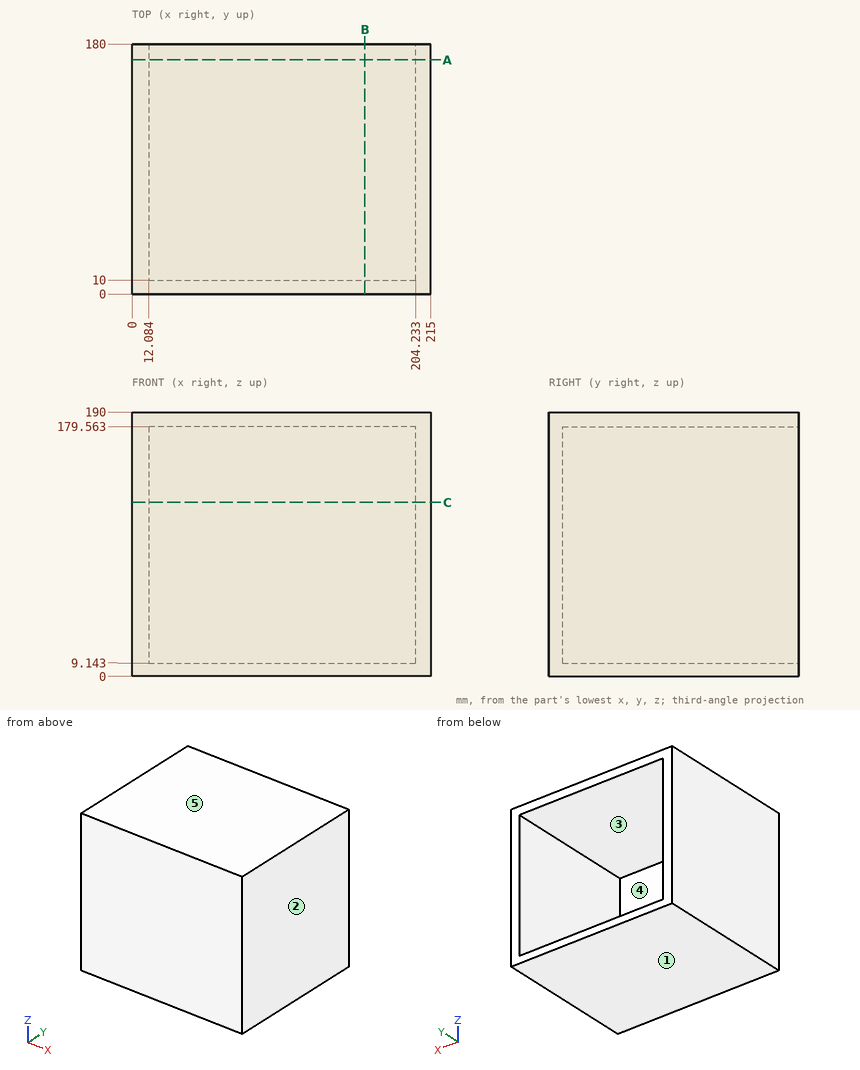
Study the drawing (mm; zero at the part's minimum x, y, z) and answer. A direction names the side the tool comes from. Round coordinates to 2 decimals unless told otherwise and drop trailing zeros. Order: outer loops, then holes, each group sorted by start corner. A loop starts at its lowest first (then second) coordinate and runs counter-clockwise, first axis right, second up. Notation, with made-up numbers: (13.25, -23) -> (48.25, -23) arc R19 ccw to (48.25, -8) -> close; hole circle Ø5 at (73.5, -30.5). An arc over 180 degrees is marked (long way). Write each question's results on one line, items separated by ' | '. Start each with the question number.
Q1. Find section A-A (y = 168.5). Determine the outline of the cut face in (x, z) (1 decimal).
Q2. Which of the six approach directions +Z, -Z, +X, -X, +Y, -Y give full straight-line access (tool end or side, diameter ignored) to the marked faces 4 and 5?
Q3. The mould has two halves that part along X. Classify the marked faces 1, 2 and 3: pulls with the +X half, pulls with the -X half, needs draft (parallel to the pull), parting line crosses it, or undercut.
Q4. Straight lines are drawn through the part: probe 1 along Z at (x, y) = (104, 119.5); probe 2 along X at (y, z) = (131.5, 48) (1 decimal); probe 3 along Y at (x, z) = (167, 87). For each, find the intervals that lie inside material, in ascending order. Write a range as from..to.
Q5. This flat-tipped pin is pushed along its axis until it touches: pin 1 (6 mm diameter, centred on x = 105, z = 167, fed in from +Y). Where does it stop, or does it pass through?
Q6. Find section B-B (x = 167.5). Determine the outline of the cut face in (y, z).
Q7. Find section C-C (z = 125). Determine the outline of the cut face in (x, y) (1 decimal).
Worked answers:
1) outline: (0, 0) -> (215, 0) -> (215, 190) -> (0, 190) -> close; hole (12.1, 9.1) -> (204.2, 9.1) -> (204.2, 179.6) -> (12.1, 179.6) -> close
2) face 4: +Y | face 5: +Z, +X, -X, +Y, -Y
3) face 1: needs draft | face 2: pulls with the +X half | face 3: undercut
4) probe 1: z = 0..9.14, 179.56..190 | probe 2: x = 0..12.1, 204.2..215 | probe 3: y = 0..10
5) pin 1: stops at y = 10
6) outline: (0, 0) -> (180, 0) -> (180, 9.14) -> (10, 9.14) -> (10, 179.56) -> (180, 179.56) -> (180, 190) -> (0, 190) -> close
7) outline: (0, 0) -> (215, 0) -> (215, 180) -> (204.2, 180) -> (204.2, 10) -> (12.1, 10) -> (12.1, 180) -> (0, 180) -> close
